Design review of the part built by this model. Coordinates are the model's own, in mm. A direction names the side the tool comes from. Coordinates: 2 decimals unless noted, no trailing zeros. Write each loop counter-clockwise with the first axis right and the second up, starting at its lowest first coordinate (ties: lowest second). Pieces come first, ordered by that corner, then holes. Notation, with made-up numbers: (85.25, 13.25) - (143.25, 13.25) arc R30 ccw to (143.25, 46.25) - close; hole circle Ø11 at (-5.75, -19.5). An arc over 180 degrees is marked (long way). Answer as a JSON object with one key per item and string values.
```python
from build123d import *

# Parameters (mm, degrees)
BOSS_EXTRUDE1_DEPTH = 25.4
BOSS_EXTRUDE2_REACH = 29.203
SKETCH5_R           = 6.9342
CUT_EXTRUDE1_DEPTH  = 25.4
CUT_EXTRUDE2_START  = -12.7
SKETCH6_R           = 6.9342
CUT_EXTRUDE2_DEPTH  = 12.7


with BuildPart() as part:
    # Sketch1 → Revolve1 (revolve)
    with BuildSketch(Plane.XY):
        Polygon((-35.052, -14.5034), (-12.7, -14.5034), (-12.7, -10.6172), (-35.052, -10.7696), align=None)
    revolve(axis=Axis((-35.052, 0, 0), (1, 0, 0)))


with BuildPart() as body_2:
    # Mirror1: mirrored copy
    add(part.part.mirror(Plane(origin=(0, 0, 0), x_dir=(0, 0, 1), z_dir=(1, 0, 0))))


with BuildPart() as body_3:
    # Sketch2 → Revolve2 (revolve)
    with BuildSketch(Plane.XY):
        Polygon((10.7696, 35.052), (10.6172, 12.7), (14.5034, 12.7), (14.5034, 35.052), align=None)
    revolve(axis=Axis((0, 0, 0), (0, 1, 0)))


with BuildPart() as part_1:
    add(part.part)

    add(body_2.part)  # Boss-Extrude1 merges body 2

    add(body_3.part)  # Boss-Extrude1 merges body 3
    # Sketch3 → Boss-Extrude1 (add)
    with BuildSketch(Plane(origin=(-12.7, 0, 0), x_dir=(0, 0, -1), z_dir=(1, 0, 0))):
        with BuildLine():
            Line((7.004185289, 12.7), (-7.004185289, 12.7))
            ThreePointArc((-7.004185289, 12.7), (0, -14.5034), (7.004185289, 12.7))
        make_face()
    extrude(amount=BOSS_EXTRUDE1_DEPTH)

    # Sketch4 → Boss-Extrude2 (add, up to next)
    with BuildSketch(Plane.XZ.offset(-12.7), mode=Mode.PRIVATE) as boss_extrude2_sk1:
        with BuildLine():
            ThreePointArc((-12.7, -7.004185289), (0, -14.5034), (12.7, -7.004185289))
            Line((12.7, -7.004185289), (-12.7, -7.004185289))
        make_face()
    boss_extrude2_tool1 = extrude(boss_extrude2_sk1.sketch, amount=BOSS_EXTRUDE2_REACH, mode=Mode.PRIVATE) - part_1.part
    add(boss_extrude2_tool1.solids().sort_by_distance((0, 12.7, -10.082201))[0])
    # Sketch4 → Boss-Extrude2 (add, up to next)
    with BuildSketch(Plane.XZ.offset(-12.7), mode=Mode.PRIVATE) as boss_extrude2_sk2:
        with BuildLine():
            ThreePointArc((12.7, 7.004185289), (0, 14.5034), (-12.7, 7.004185289))
            Line((-12.7, 7.004185289), (12.7, 7.004185289))
        make_face()
    boss_extrude2_tool2 = extrude(boss_extrude2_sk2.sketch, amount=BOSS_EXTRUDE2_REACH, mode=Mode.PRIVATE) - part_1.part
    add(boss_extrude2_tool2.solids().sort_by_distance((0, 12.7, 10.082201))[0])

    # Sketch5 → Cut-Extrude1 (cut)
    with BuildSketch(Plane.ZY.offset(12.7)):
        Circle(SKETCH5_R)
    extrude(amount=-CUT_EXTRUDE1_DEPTH, mode=Mode.SUBTRACT)

    # Sketch6 → Cut-Extrude2 (cut)
    with BuildSketch(Plane(origin=(0, 12.7, 0), x_dir=(1, 0, 0), z_dir=(0, 1, 0)).offset(CUT_EXTRUDE2_START)):
        Circle(SKETCH6_R)
    extrude(amount=CUT_EXTRUDE2_DEPTH, mode=Mode.SUBTRACT)


solid = part_1.part
```
(1) Take a section at C-C, the plane x = -19.5. Write out the cut boundary in (y, z).
Solved:
{"outline": "circle Ø29.01 at (0, 0); hole circle Ø21.33 at (0, 0)"}
(2) The part is to be moulded in two halves that separate along Y. For faces 1 (the face through (-35.052, 0, -11)), 2 (the face through (-12.7, -7, -2)), 3 (the face through (-2.318, 23.72, 10.438)), say which applies: pulls with the +Y half, pulls with the -Y half, needs draft (parallel to the pull), parting line crosses it, or undercut.
Solved:
{"face 1": "needs draft", "face 2": "undercut", "face 3": "pulls with the +Y half"}
(3) For pin 1 (2 mm diameter, centred on y = 28.5, z = 11, fed in from +X); pin 2 (8 mm diameter, centred on y = 14, z = 8.5, fed in from -X); pin 3 (8 mm diameter, centred on x = 11, y = 4.5, fed in from -Z); pin 4 (8.5 mm diameter, centred on x = 0, z = 0, fed in from +Y), all flat-tipped, find the tip position at first contact; note any pin that passes through.
Solved:
{"pin 1": "stops at x = 10.5", "pin 2": "stops at x = -35.05", "pin 3": "stops at z = -14.49", "pin 4": "stops at y = -5.48"}
(4) Tool access review of faces 4 (the face through (35.052, 0, -11)), 5 (the face through (-0.18, -6.77, -1.5)), 6 (the face through (-24.03, -10.2, -3.21)), 7 (the face through (-1.5, 7.67, 6.77)), 8 (the face through (24.03, -10.2, -3.21)): name each direction out of +Z, -Z, +X, -X, +Y, -Y from which nothing blocks a thin tool from reaching the whole face with its end or side.
Solved:
{"face 4": "+Z, -Z, +X, +Y, -Y", "face 5": "+X, -X", "face 6": "-X", "face 7": "+Y", "face 8": "+X"}
(5) To check wall thickness, follow line 1 (Z direction, x = -0.25, y = 0); line 2 (X direction, y = 7, z = 0); line 3 (Z direction, x = 21.5, y = -7.5). State the ranges of each line that lie inside material, in increasing order. Write a range as from..to.
Solved:
{"line 1": "z = -14.5..-6.93, 6.93..14.5", "line 2": "x = -12.7..-6.93, 6.93..12.7", "line 3": "z = -12.41..-7.6, 7.6..12.41"}
(6) Take a section at B-B, the plane z = 12. Write out the cut boundary in (x, y).
Solved:
{"outline": "(-35.05, -8.15) - (35.05, -8.15) - (35.05, 8.15) - (8.15, 8.15) - (8.15, 35.05) - (-8.15, 35.05) - (-8.15, 8.15) - (-35.05, 8.15) - close"}
(7) Take a section at D-D, the plane y = 26. Write out the cut boundary in (x, z), and give its area (3 significant figures).
Solved:
{"outline": "circle Ø29.01 at (0, 0); hole circle Ø21.42 at (0, 0)", "area": "301 mm^2"}
(8) Take a section at A-A, the plane z = 0. Give the number of separate pieces and of enclosed holes in the cut face, and give its area (3 significant figures).
Solved:
{"separate pieces": "3", "enclosed holes": "0", "area": "763 mm^2"}
